Here's the drawing with two shaded views (mm, measured from the low corner). I have some questions. Give positions to 0.01 mm unless a question says otherwise; leave off trailing zeros. Write each loop counter-clockwise with the first axis right and the second up, starting at its lowest first coordinate (ties: lowest second). Pieces come first, ordered by that corner, then holes. Notation, with made-up numbers: (46, 81.5) - (76, 81.5) arc R32 ccw to (76, 118.5) - close; hole circle Ø5 at (-2, 37). An arc over 180 degrees is marked (long way). Answer as CSV lines item,"result". Start each with the question number.
Q1. Imagine slicing it at B-B on z = 6.35. List the corners of the cut face in (x, y) for me.
Q2. Will these pins go through, and if not, where does the flat tip stop? pin 1 Ø1.1 at (x, y) = (3, 1.5) entering from +Z; pin 2 Ø1.8 at (x, z) = (9.65, 6.35) entering from -Y; pin 3 Ø0.7 at (x, z) = (11.5, 8.5) entering from +Y; pin 4 Ø0.5 at (x, z) = (6.5, 8.5) entering from -Y.
Q3. Imagine slicing it at C-C on y = 0.65. List the corners of the cut face in (x, z) for me.
Q4. Imagine slicing it at D-D on x = 7.5. List the corners of the cut face in (y, z) for me.
Q5. We'd pull the mould along Z, two halves only. Please class the marked faces 1, 2 and 3: pulls with the +Z half, pulls with the -Z half, needs draft (parallel to the pull), parting line crosses it, or undercut.
Q6. Imagine slicing it at A-A on x = 3.15. List the corners of the cut face in (y, z) for me, and give its area (3 significant figures).
Q7. If I drill on line 1 along X through (y, z) = (2.9, 6.35); line 2 along Z through (x, y) = (9.65, 3.1); line 3 along X through (y, z) = (2.95, 7.5), over which ranges is the centre line in solid material (lowest first)?
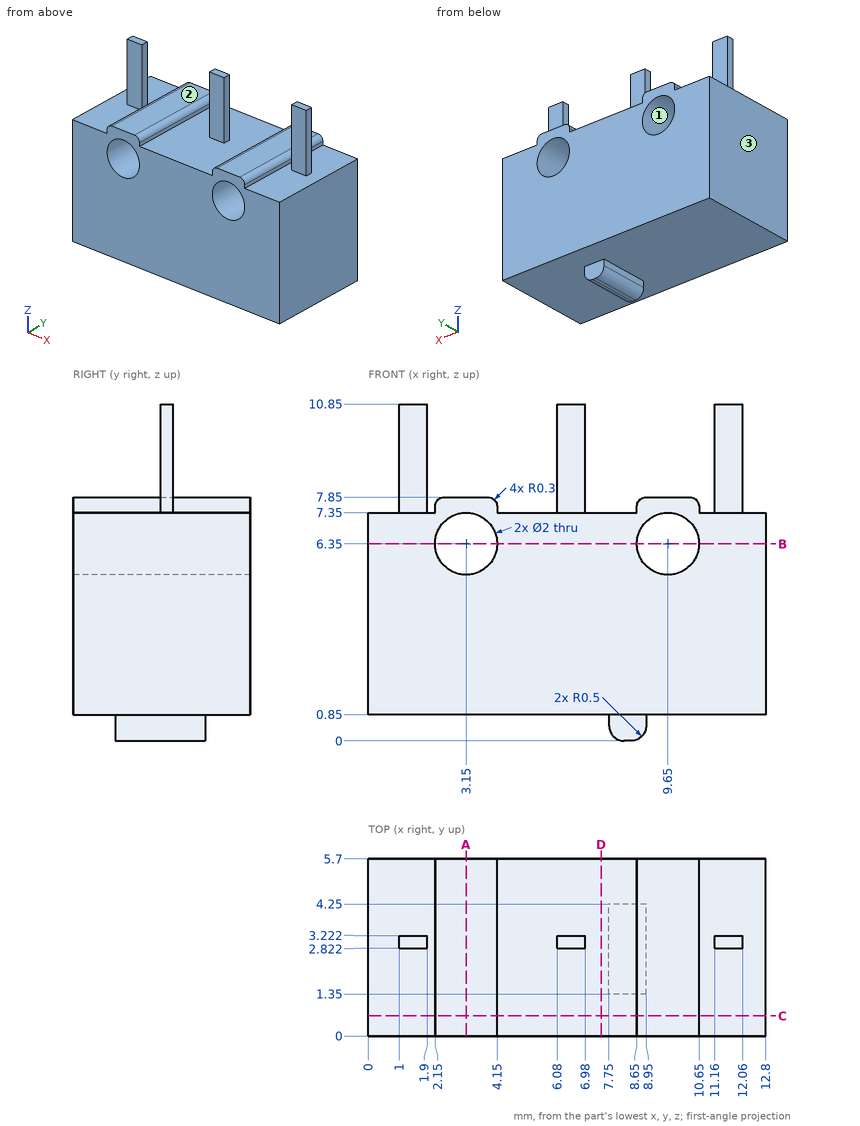
Conclusion:
1,outline,"(0, 0) - (2.15, 0) - (2.15, 5.7) - (0, 5.7) - close; (4.15, 0) - (8.65, 0) - (8.65, 5.7) - (4.15, 5.7) - close; (10.65, 0) - (12.8, 0) - (12.8, 5.7) - (10.65, 5.7) - close"
2,pin 1,"z = 7.85"
2,pin 2,"through"
2,pin 3,"y = 3.22"
2,pin 4,"y = 2.82"
3,outline,"(0, 0.85) - (12.8, 0.85) - (12.8, 7.35) - (10.65, 7.35) - (10.65, 7.55) arc R0.3 ccw to (10.35, 7.85) - (8.95, 7.85) arc R0.3 ccw to (8.65, 7.55) - (8.65, 7.35) - (4.15, 7.35) - (4.15, 7.55) arc R0.3 ccw to (3.85, 7.85) - (2.45, 7.85) arc R0.3 ccw to (2.15, 7.55) - (2.15, 7.35) - (0, 7.35) - close; hole circle Ø2 at (3.15, 6.35); hole circle Ø2 at (9.65, 6.35)"
4,outline,"(0, 0.85) - (5.7, 0.85) - (5.7, 7.35) - (0, 7.35) - close"
5,face 1,"undercut"
5,face 2,"pulls with the +Z half"
5,face 3,"needs draft"
6,outline,"(0, 0.85) - (5.7, 0.85) - (5.7, 5.35) - (0, 5.35) - close; (0, 7.35) - (5.7, 7.35) - (5.7, 7.85) - (0, 7.85) - close"
6,area,"28.5 mm^2"
7,line 1,"0 to 2.15, 4.15 to 8.65, 10.65 to 12.8"
7,line 2,"0.85 to 5.35, 7.35 to 7.85"
7,line 3,"1 to 1.9, 2.15 to 4.15, 6.08 to 6.98, 8.65 to 10.65, 11.16 to 12.06"
